For this review, take the finished solid that the model builds, in its own axes (mm). Face numbers are marked on the shaded views. A direction names the side the tool comes from. Give positions to 0.01 mm unless a question says otherwise; leave off trailing zeros. Order: outer loops, then holes, each group sorted by start corner. A loop starts at its lowest first (then second) coordinate and runs counter-clockwise, first axis right, second up. Notation, with made-up numbers: (56.5, -38) -> (81.5, -38) arc R27 ccw to (81.5, -13) -> close; hole circle Ø10 at (63, -26.75). An arc over 180 degrees is marked (long way). Return JSON: item names as keys, results as strings. Group by question number.
1) To check wall thickness, follow line 1 along Y through (x, z) = (-6.5, -5); line 2 along Z through (x, y) = (27.5, -4); line 3 along Y through (x, z) = (10, 29.5). State the ranges of each line that lie inside material, in increasing order.
2) Insertion check: P1, Ø2.5, axis at x = -23, y = -1.5, coming from the +Z side; P2, Ø4, axis at y = 1, z = 19, coming from the -X side; P3, Ø2.5, axis at y = 0.5, z = -19.5, coming from the +X side. Each pin has a flat end and moves straight along its axis. Give the tip position at first contact, or say it passes through.
3) Add section C-C (z = -9). Give the boundary of the cut face in (x, y).
4) For the marked faces 1, 2, 3 and 4, list the 3-axis set-ups (+Z, -Z, +X, -X, +Y, -Y) from which the entire face can be reached by the end or side of a thin tool; tool diameter is ignored.
5) Add section B-B (x = -4.5). Give the boundary of the cut face in (y, z).
6) Add section D-D (z = 3). Give the boundary of the cut face in (x, y), then the cut area to 3 significant figures.
7) Add section A-A (y = -3). Give the boundary of the cut face in (x, z), then the cut area to 3 significant figures.
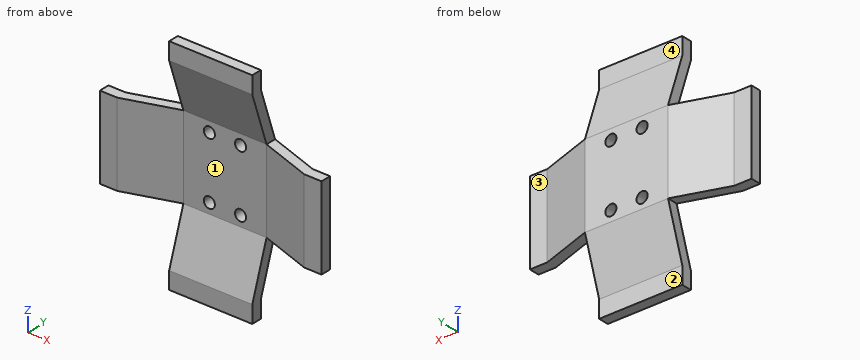
Autodesk Fusion 360 part; units mm, degrees
sketch "スケッチ1" plane through (0, 0, 0) normal (0, 1, 0) x (1, 0, 0)
  line L0 (12, 12) -> (-12, 12)
  line L1 (-12, 12) -> (-12, -12)
  line L2 (-12, -12) -> (12, -12)
  line L3 (12, -12) -> (12, 12)
  line L4 (12, 12) -> (-12, -12) construction
  line L5 (-12, 12) -> (12, -12) construction
  line L6 (4.5, 9) -> (-4.5, 9)
  line L7 (-4.5, 9) -> (-4.5, -9)
  line L8 (-4.5, -9) -> (4.5, -9)
  line L9 (4.5, -9) -> (4.5, 9)
  line L10 (4.5, 9) -> (-4.5, -9) construction
  line L11 (-4.5, 9) -> (4.5, -9) construction
  circle A0 centre (-4.5, 9) radius 1.6
  circle A1 centre (4.5, 9) radius 1.6
  circle A2 centre (-4.5, -9) radius 1.6
  circle A3 centre (4.5, -9) radius 1.6
  dimension "d1" = 24
  dimension "d2" = 24
  dimension "d3" = 9
  dimension "d4" = 18
  dimension "d5" = 3.2
  dimension "d6" = 3.2
  dimension "d7" = 3.2
  dimension "d8" = 3.2
extrude "押し出し1" add sketch "スケッチ1" along normal blind 3 contours L0 L1 L2 L3 | L6 L7 L8 L9 A0 A1 A2 A3
sketch "スケッチ2" plane through (0, 0, 0) normal (0, 0, 1) x (1, 0, 0)
  line L0 (12, 0) -> (12, -5)
  line L1 (12, -5) -> (27, -5)
  line L2 (27, -5) -> (12, 0)
  line L3 (27, -5) -> (27, -2)
  line L4 (27, -2) -> (12, 3)
  line L5 (12, 0) -> (12, 3)
  line L6 (27, -2) -> (32, -2)
  line L7 (32, -2) -> (32, -5)
  line L8 (32, -5) -> (27, -5)
  line L9 (27, -5) -> (27, -2)
  dimension "d11" = 5
  dimension "d12" = 15
  dimension "d13" = 3
  dimension "d14" = 5
  dimension "d15" = 3
extrude "押し出し2" add sketch "スケッチ2" along normal mid plane 24 contours L2 L3 L4 L5 L9 | L3 L6 L7 L8 L9
sketch "スケッチ3" plane through (0, 0, 0) normal (0, 0, 1) x (1, 0, 0)
  line L0 (-12, 0) -> (-12, -5)
  line L1 (-12, -5) -> (-27, -5)
  line L2 (-12, 0) -> (-27, -5)
  line L3 (-27, -5) -> (-27, -2)
  line L4 (-27, -2) -> (-12, 3)
  line L5 (-12, 3) -> (-12, 0)
  line L6 (-27, -2) -> (-32, -2)
  line L7 (-32, -2) -> (-32, -5)
  line L8 (-32, -5) -> (-27, -5)
  line L9 (-27, -5) -> (-27, -2)
  dimension "d18" = 5
  dimension "d19" = 15
  dimension "d20" = 3
  dimension "d21" = 5
  dimension "d22" = 3
extrude "押し出し3" add sketch "スケッチ3" along normal mid plane 24 contours L2 L3 L4 L5 L9 | L3 L6 L7 L8 L9
sketch "スケッチ4" plane through (0, 0, 0) normal (1, 0, 0) x (0, 0, -1)
  line L0 (12, 0) -> (12, -5)
  line L1 (12, -5) -> (27, -5)
  line L2 (27, -5) -> (12, 0)
  line L3 (27, -5) -> (27, -2)
  line L4 (27, -2) -> (12, 3)
  line L5 (12, 3) -> (12, 0)
  line L6 (27, -2) -> (32, -2)
  line L7 (32, -2) -> (32, -5)
  line L8 (32, -5) -> (27, -5)
  line L9 (27, -5) -> (27, -2)
  line L10 (0, 5) -> (0, 4)
  line L11 (0, 4) -> (0, -9)
  line L12 (-27, -2) -> (-12, 3)
  line L13 (-12, 3) -> (-12, 0)
  line L14 (-27, -5) -> (-12, 0)
  line L15 (-27, -2) -> (-32, -2)
  line L16 (-27, -5) -> (-27, -2)
  line L17 (-32, -2) -> (-32, -5)
  line L18 (-32, -5) -> (-27, -5)
  dimension "d25" = 15
  dimension "d26" = 3
  dimension "d27" = 3
  dimension "d28" = 5
extrude "押し出し4" add sketch "スケッチ4" along normal mid plane 24 contours L2 L3 L4 L5 L9 | L3 L6 L7 L8 L9 | L15 L16 L17 L18 | L12 L13 L14 L16
Evaluation:
{
 "1": {"line 1": "0 to 3", "line 2": "-12 to 12", "line 3": "-5 to -2"},
 "2": {"P1": "z = 12", "P2": "x = -12", "P3": "x = 12"},
 "3": {"outline": "(-32, -5) -> (-27, -5) -> (-12, 0) -> (-6.1, 0) -> (-6.1, 3) -> (-12, 3) -> (-27, -2) -> (-32, -2) -> close; (-2.9, 0) -> (2.9, 0) -> (2.9, 3) -> (-2.9, 3) -> close; (6.1, 0) -> (12, 0) -> (27, -5) -> (32, -5) -> (32, -2) -> (27, -2) -> (12, 3) -> (6.1, 3) -> close"},
 "4": {"face 1": "-Y", "face 2": "-Z, +X, -X, +Y", "face 3": "+Z, -Z, +X, +Y", "face 4": "+Z, +X, -X, +Y"},
 "5": {"outline": "(-5, -32) -> (-2, -32) -> (-2, -27) -> (3, -12) -> (3, -10.6) -> (0, -10.6) -> (0, -12) -> (-5, -27) -> close; (-5, 27) -> (0, 12) -> (0, 10.6) -> (3, 10.6) -> (3, 12) -> (-2, 27) -> (-2, 32) -> (-5, 32) -> close; (0, -7.4) -> (3, -7.4) -> (3, 7.4) -> (0, 7.4) -> close"},
 "6": {"outline": "(-32, -5) -> (-27, -5) -> (-12, 0) -> (12, 0) -> (27, -5) -> (32, -5) -> (32, -2) -> (27, -2) -> (12, 3) -> (-12, 3) -> (-27, -2) -> (-32, -2) -> close", "area": "192 mm^2"},
 "7": {"outline": "(-32, -12) -> (-21, -12) -> (-21, 12) -> (-32, 12) -> close; (-12, -32) -> (12, -32) -> (12, -21) -> (-12, -21) -> close; (-12, 21) -> (12, 21) -> (12, 32) -> (-12, 32) -> close; (21, -12) -> (32, -12) -> (32, 12) -> (21, 12) -> close", "area": "1,060 mm^2"}
}
